The drawing under review shows one solid part. Ordinate dimensions are in mm from its lowest x, y, z. A direction names the side the tool comes from. Coordinates: 2 decimals unless noted, no trailing zeros. Order: outer loops, then holes, each group sorted by start corner. A loop starts at its lowest first (then second) coordinate and runs counter-clockwise, first axis right, second up.
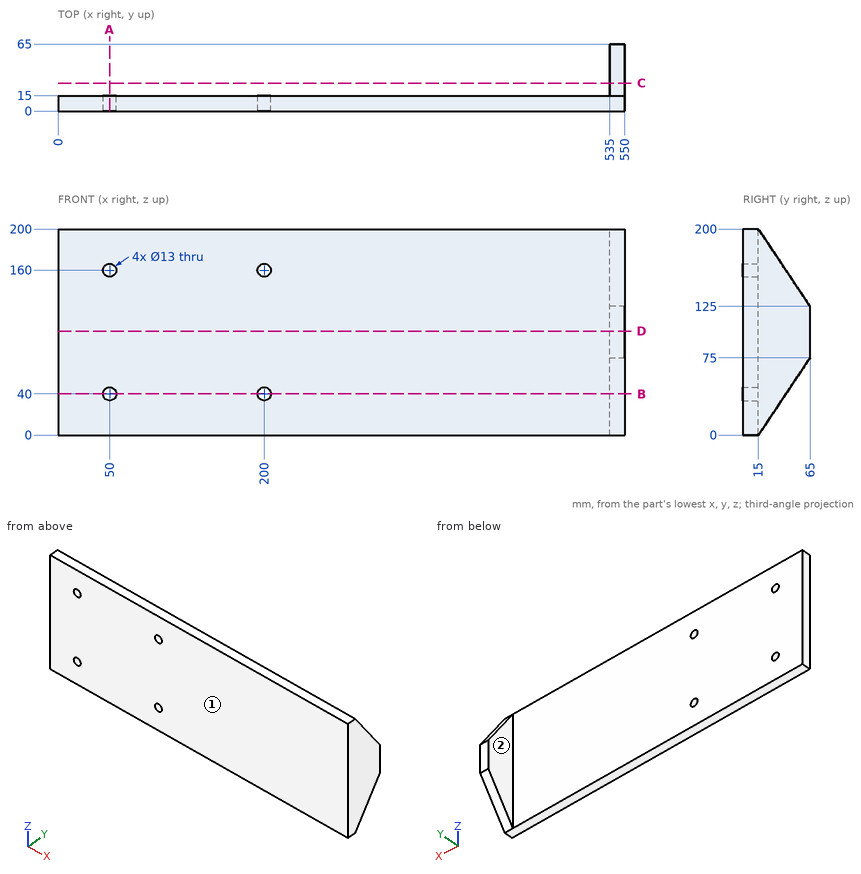
(1) We need section D-D, the plane z = 101. Write out the cut boundary in (x, y), and give its area (3 significant figures).
A:
outline: (0, 0) - (550, 0) - (550, 65) - (535, 65) - (535, 15) - (0, 15) - close
area: 9,000 mm2
(2) We need section C-C, the plane y = 27. Write out the cut boundary in (x, z).
A:
outline: (535, 18) - (550, 18) - (550, 182) - (535, 182) - close
(3) For pin 1 Ø11.5 at (x, z) = (200, 40) entering from +Y; pin 2 Ø8 at (y, z) = (50, 86) entering from -X; pin 3 Ø15 at (x, z) = (50, 160) entering from +Y, all flat-tipped, find the tip position at first contact; note any pin that passes through.
A:
pin 1: passes through
pin 2: stops at x = 535
pin 3: stops at y = 15
(4) We need section B-B, the plane z = 40. Write out the cut boundary in (x, y).
A:
outline: (0, 0) - (43.5, 0) - (43.5, 15) - (0, 15) - close; (56.5, 0) - (193.5, 0) - (193.5, 15) - (56.5, 15) - close; (206.5, 0) - (550, 0) - (550, 41.67) - (535, 41.67) - (535, 15) - (206.5, 15) - close
(5) We need section A-A, the plane x = 50. Write out the cut boundary in (y, z).
A:
outline: (0, 0) - (15, 0) - (15, 33.5) - (0, 33.5) - close; (0, 46.5) - (15, 46.5) - (15, 153.5) - (0, 153.5) - close; (0, 166.5) - (15, 166.5) - (15, 200) - (0, 200) - close
(6) Wall thickness on probe 1 along Z at (x, y) = (50, 11); probe 2 along X at (y, z) = (10, 160.5); probe 3 along Y at (x, z) = (407.5, 191.5): over which ranges is each line inside the solid? List them lowest first.
A:
probe 1: z = 0 to 33.5, 46.5 to 153.5, 166.5 to 200
probe 2: x = 0 to 43.52, 56.48 to 193.52, 206.48 to 550
probe 3: y = 0 to 15
(7) Machinability: for the marked faces 1 and 2, which of the approach directions +Z, -Z, +X, -X, +Y, -Y give a long, thin tool a straight path to every point of the face, cutting with its end or side? Answer none if there is none.
A:
face 1: +Z, -Z, +X, -X, -Y
face 2: +Z, -Z, -X, +Y
